from build123d import *

# Parameters (mm, degrees)
F1_DEPTH = 250
F2_DEPTH = 125


with BuildPart() as f1:
    # F0 (on Front) → F1 (new body, symmetric)
    with BuildSketch(Plane.XZ):
        with BuildLine():
            Line((-14.503544, 3.604437), (-13.457058, 6.465255))
            ThreePointArc((-13.457058, 6.465255), (-55.63549, 10.165767), (-97.795863, 6.264893))
            Line((-97.795863, 6.264893), (-97.003544, 3.360226))
            ThreePointArc((-97.003544, 3.360226), (-55.764447, 7.165413), (-14.503544, 3.604437))
        make_face()
    extrude(amount=F1_DEPTH, both=True)

    # F0 (on Front) → F2 (join, symmetric)
    with BuildSketch(Plane.XZ):
        with BuildLine():
            Line((12.996456, -3.006309), (14.042942, -0.189243))
            ThreePointArc((14.042942, -0.189243), (0.392824, 3.550775), (-13.457058, 6.465255))
            Line((-13.457058, 6.465255), (-14.503544, 3.604437))
            ThreePointArc((-14.503544, 3.604437), (-0.653074, 0.717009), (12.996456, -3.006309))
        make_face()
    extrude(amount=F2_DEPTH, both=True)


solid = f1.part
Verification items for the finished model (mm, model axes). Coordinates: 2 decimals unless noted, no trailing zeros. Order: outer loops, then holes, each group sorted by start corner. A loop starts at its lowest first (then second) coordinate and runs counter-clockwise, first axis right, second up. Notation, with made-up numbers: M 64.25,17.25 L 79.25,17.25 A5 ccw 79.25,22.25 Z; hole C 54.25,-32 d10. An arc over 180 degrees is marked long. Return JSON: item names as keys, results as strings.
1) Cross-section at C-C, the plane y = 140. Record the boundary of the cut face in (x, z).
Answer list:
{"outline": "M -97.8,6.26 L -97,3.36 A232.84 cw -14.5,3.6 L -13.46,6.47 A235.84 ccw Z"}
2) Thickness scan on L1, parallel to Z at x = -52, y = 34.5; L2, parallel to Y at x = -1.5, z = 2; L3, parallel to Z at x = -56.5, y = 111.5. Record the ranges inside material, lowest first. Write a range as [from, to].
Answer list:
{"L1": "[7.15, 10.15]", "L2": "[-125, 125]", "L3": "[7.16, 10.16]"}
3) Release check for a two-part mould opening along X. For faces 1 (the cylindrical face through (-0.846, -1.75, 0.763)), 2 (the cylindrical face through (-56.345, -3.5, 7.163)), 3 (the flat face through (0, 125, 2)) record: +X half, -X half, draft (parallel to the pull), parting line (faces both ways), or undercut.
Answer list:
{"face 1": "-X half", "face 2": "undercut", "face 3": "draft"}
4) Cross-section at A-A, the plane y = -40. Record the boundary of the cut face in (x, z), and give its area (3 significant figures).
Answer list:
{"outline": "M -97.8,6.26 L -97,3.36 A232.84 cw -14.5,3.6 A232.84 cw 13,-3.01 L 14.04,-0.19 A235.84 ccw -13.46,6.47 A235.84 ccw Z", "area": "337 mm2"}
5) Cross-section at B-B, the plane x = -57.5. Record the boundary of the cut face in (y, z).
Answer list:
{"outline": "M -250,7.15 L 250,7.15 L 250,10.15 L -250,10.15 Z"}
6) Gauge pin test, flat ends, axial feed: pin 1 (3 mm diameter, centred on x = -6.5, z = -0.5, fed in from -Y); pin 2 (1 mm diameter, centred on x = -41, y = -121.5, fed in from +Z); pin 3 (2 mm diameter, centred on x = -29, y = 136, fed in from +Z). Record the tip position at first contact, or that the pin passes through.
Answer list:
{"pin 1": "through", "pin 2": "z = 9.78", "pin 3": "z = 8.83"}
